The drawing under review shows one solid part. Ordinate dimensions are in mm from its lowest x, y, z. Give positions to 0.01 mm unless a question says otherwise; leave off trailing zeros. Order: outer loops, then holes, each group sorted by start corner. A loop starts at its lowest first (then second) coordinate and runs counter-clockwise, first axis right, second up. Notation, with made-up numbers: M 26.5,-35 L 39.5,-35 A27 ccw 39.5,-9 Z; hole C 87,80 d11. An arc over 180 degrees is marked long. Put each result on its own line as item: value. Start each with the question number.
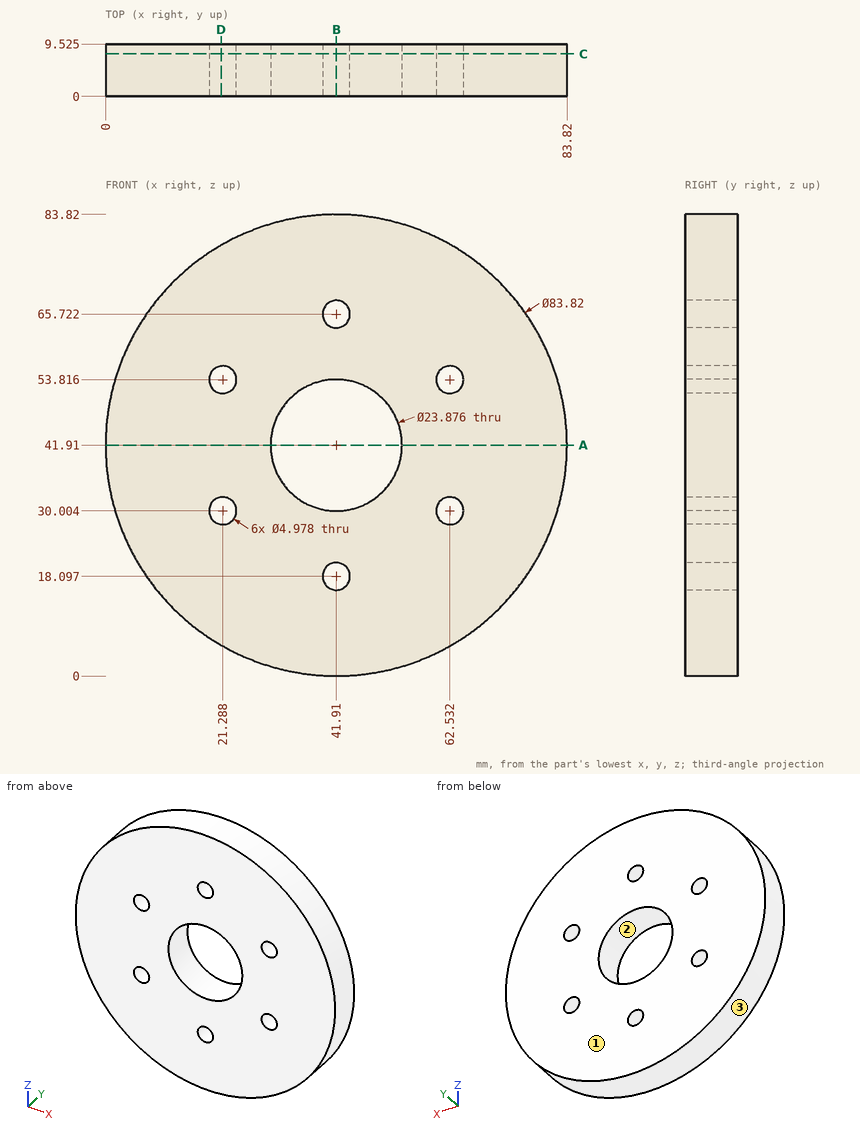
1. Consider section C-C on y = 7.75. Give the boundary of the cut face in (x, z) (1 decimal).
2. Consider section B-B on x = 41.91. Give the boundary of the cut face in (y, z) (1 decimal), then the cut area to 3 significant figures.
3. The part is to be moulded in two halves that separate along Z. For the marked faces 1, 2 and 3, say which applies: +Z half, -Z half, draft (parallel to the pull), parting line (faces both ways), or undercut.
4. To check wall thickness, follow probe 1 along Z at (x, y) = (41.91, 3); probe 2 along Z at (x, y) = (21, 4.75) (1 decimal); probe 3 along Z at (x, y) = (45, 6.5) (1 decimal). State the ranges of each line that lie inside material, in increasing order.
5. Consider section A-A on z = 41.91. Give the boundary of the cut face in (x, y) (1 decimal), then the cut area to 3 significant figures.
6. Insertion check: pin 1 (5 mm diameter, centred on x = 27.5, y = 7.5, fed in from +Z); pin 2 (10 mm diameter, centred on x = 54, z = 34.5, fed in from -Y); pin 3 (1 mm diameter, centred on y = 3, z = 28, fed in from -X); pin 4 (3 mm diameter, centred on x = 46.5, y = 3, fed in from -Z). Each pin has a flat end and moves straight along its axis. Give the tip position at first contact, or say it passes through.
7. Consider section D-D on x = 21. Give the boundary of the cut face in (y, z) (1 decimal).
Returned:
1. outline: C 41.9,41.9 d83.8; hole C 21.3,30 d5; hole C 21.3,53.8 d5; hole C 41.9,41.9 d23.9; hole C 41.9,18.1 d5; hole C 41.9,65.7 d5; hole C 62.5,30 d5; hole C 62.5,53.8 d5
2. outline: M 0,0 L 9.5,0 L 9.5,15.6 L 0,15.6 Z; M 0,20.6 L 9.5,20.6 L 9.5,30 L 0,30 Z; M 0,53.8 L 9.5,53.8 L 9.5,63.2 L 0,63.2 Z; M 0,68.2 L 9.5,68.2 L 9.5,83.8 L 0,83.8 Z
2. area: 476 mm2
3. face 1: draft
3. face 2: undercut
3. face 3: parting line
4. probe 1: z = 0 to 15.61, 20.59 to 29.97, 53.85 to 63.23, 68.21 to 83.82
4. probe 2: z = 5.6 to 27.5, 32.5 to 51.3, 56.3 to 78.2
4. probe 3: z = 0.1 to 30.4, 53.4 to 83.7
5. outline: M 0,0 L 30,0 L 30,9.5 L 0,9.5 Z; M 53.8,0 L 83.8,0 L 83.8,9.5 L 53.8,9.5 Z
5. area: 571 mm2
6. pin 1: stops at z = 82.09
6. pin 2: stops at y = 0
6. pin 3: stops at x = 2.2
6. pin 4: stops at z = 0.11
7. outline: M 0,5.6 L 9.5,5.6 L 9.5,27.5 L 0,27.5 Z; M 0,32.5 L 9.5,32.5 L 9.5,51.3 L 0,51.3 Z; M 0,56.3 L 9.5,56.3 L 9.5,78.2 L 0,78.2 Z
